```python
from build123d import *

# Parameters (mm, degrees)
SKETCH_1_W      = 68
SKETCH_1_H      = 38
SKETCH_1_R      = 1.5
SKETCH_1_R_2    = 2.5
EXTRUDE_1_DEPTH = 3
SKETCH_2_R      = 4
SKETCH_2_R_2    = 1.5
EXTRUDE_2_DEPTH = 19
FILLET_1_R      = 4


with BuildPart() as part:
    # 草图1 → 凸台-拉伸1 (new body)
    with BuildSketch(Plane(origin=(0, 0, 0), x_dir=(1, 0, 0), z_dir=(0, 1, 0))):
        with Locations((10, -0.865384615)):
            Rectangle(SKETCH_1_W, SKETCH_1_H)
        with Locations(Location((-20, -15.865384615, 0), (0, 0, 270))):
            Circle(SKETCH_1_R, mode=Mode.SUBTRACT)
        with Locations(Location((-20, 14.134615385, 0), (0, 0, 270))):
            Circle(SKETCH_1_R, mode=Mode.SUBTRACT)
        with Locations(Location((40, 14.134615385, 0), (0, 0, 270))):
            Circle(SKETCH_1_R, mode=Mode.SUBTRACT)
        with Locations(Location((40, -15.865384615, 0), (0, 0, 270))):
            Circle(SKETCH_1_R, mode=Mode.SUBTRACT)
        with Locations(Location((-17.5, -0.865384615, 0), (0, 0, 270))):
            Circle(SKETCH_1_R_2, mode=Mode.SUBTRACT)
        with Locations(Location((37.5, -0.865384615, 0), (0, 0, 90))):
            Circle(SKETCH_1_R_2, mode=Mode.SUBTRACT)
        with Locations(Location((25, 14.134615385, 0), (0, 0, 270))):
            Circle(SKETCH_1_R, mode=Mode.SUBTRACT)
    extrude(amount=EXTRUDE_1_DEPTH)

    # 草图2 → 凸台-拉伸2 (add)
    # profile 1 of 4: a face of its own
    with BuildSketch(Plane(origin=(0, 3, 0), x_dir=(1, 0, 0), z_dir=(0, 1, 0))):
        with Locations(Location((-20, -15.865384615, 0), (0, 0, 270))):
            Circle(SKETCH_2_R)
        with Locations(Location((-20, -15.865384615, 0), (0, 0, 270))):
            Circle(SKETCH_2_R_2, mode=Mode.SUBTRACT)
    # profile 2 of 4: a face of its own
    with BuildSketch(Plane(origin=(0, 3, 0), x_dir=(1, 0, 0), z_dir=(0, 1, 0))):
        with Locations(Location((40, -15.865384615, 0), (0, 0, 270))):
            Circle(SKETCH_2_R)
        with Locations(Location((40, -15.865384615, 0), (0, 0, 270))):
            Circle(SKETCH_2_R_2, mode=Mode.SUBTRACT)
    # profile 3 of 4: a face of its own
    with BuildSketch(Plane(origin=(0, 3, 0), x_dir=(1, 0, 0), z_dir=(0, 1, 0))):
        with Locations(Location((-20, 14.134615385, 0), (0, 0, 90))):
            Circle(SKETCH_2_R)
        with Locations(Location((-20, 14.134615385, 0), (0, 0, 270))):
            Circle(SKETCH_2_R_2, mode=Mode.SUBTRACT)
    # profile 4 of 4: a face of its own
    with BuildSketch(Plane(origin=(0, 3, 0), x_dir=(1, 0, 0), z_dir=(0, 1, 0))):
        with Locations(Location((40, 14.134615385, 0), (0, 0, 90))):
            Circle(SKETCH_2_R)
        with Locations(Location((40, 14.134615385, 0), (0, 0, 270))):
            Circle(SKETCH_2_R_2, mode=Mode.SUBTRACT)
    extrude(amount=EXTRUDE_2_DEPTH)

    # 圆角1
    fillet_1_edges = [part.edges().sort_by_distance(p)[0] for p in [
        (44, 1.5, 19.865384615),
        (44, 1.5, -18.134615385),
        (-24, 1.5, -18.134615385),
        (-24, 1.5, 19.865384615),
    ]]
    fillet(fillet_1_edges, radius=FILLET_1_R - 0.0001)  # a hair under: the kernel refuses the full size


solid = part.part
```
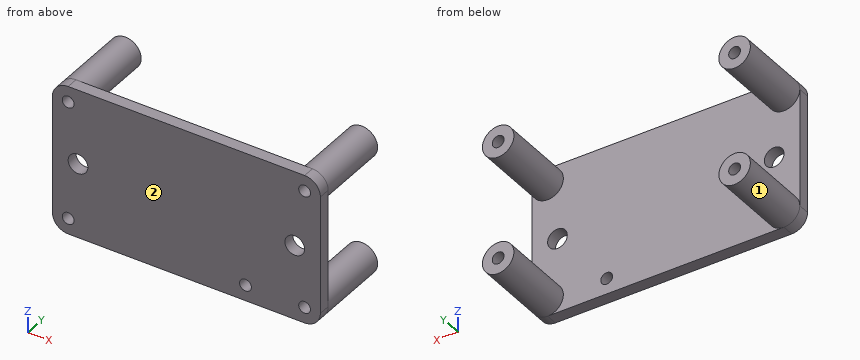
Could you check a few things on this model? Use its own coordinates, in mm. Face numbers are marked on the shaded views. Give positions to 0.01 mm unless a question says otherwise; leave off trailing zeros. Loops run counter-clockwise (first coordinate to the right, second up) from the corner with the lowest first, then second, coordinate; pieces in that order, holes last. Notation, with made-up numbers: (54.25, 84) - (93.25, 84) arc R34 ccw to (93.25, 116) - close; hole circle Ø7 at (84, -20.5). An arc over 180 degrees is marked (long way). Use one line per item in the form item = value.
1. I want a section at D-D (z = 8.5). Please give me the cut outline in (x, y), and give its area (3 significant figures).
Response values:
outline = (-24, 0) - (44, 0) - (44, 3) - (-24, 3) - close
area = 204 mm²
2. I need wall thicknesses on probe 1 along Z at (x, y) = (37.5, 1); probe 2 along Y at (x, z) = (38.5, 11.5); probe 3 along Z at (x, y) = (-18, 6.25). Which ranges of each line are inside material? Lowest first, please.
Response values:
probe_1 = -18.13 to -1.63, 3.37 to 19.87
probe_2 = 0 to 3
probe_3 = -17.6 to -10.67, 12.4 to 19.33
3. I want a section at A-A (y = 15). Please give me the cut outline in (x, z), and give its area (3 significant figures).
Response values:
outline = circle Ø8 at (-20, -14.13); circle Ø8 at (-20, 15.87); circle Ø8 at (40, -14.13); circle Ø8 at (40, 15.87); hole circle Ø3 at (-20, -14.13); hole circle Ø3 at (-20, 15.87); hole circle Ø3 at (40, -14.13); hole circle Ø3 at (40, 15.87)
area = 173 mm²
4. Thinking about a two-plate mould opening in Z: for the marked faces 1 and 2, which applies, released by +Z, released by -Z, zero draft, split by the parting line, or undercut?
Response values:
face_1 = undercut
face_2 = zero draft
5. I'm going to push flat-ended pins straight in: pin 1 Ø2.5 at (x, z) = (40, 15.87) entering from +Y; pin 2 Ø11.5 at (x, z) = (19, 6.5) entering from +Y. Where does each tip first touch, or does it pass through?
Response values:
pin_1 = through
pin_2 = 3
6. I want a section at B-B (x = 25). Please give me the cut outline in (y, z), and give its area (3 significant figures).
Response values:
outline = (0, -18.13) - (3, -18.13) - (3, -15.63) - (0, -15.63) - close; (0, -12.63) - (3, -12.63) - (3, 19.87) - (0, 19.87) - close
area = 105 mm²
7. I want a section at C-C (z = -0.5). Please give me the cut outline in (x, y).
Response values:
outline = (-24, 0) - (-19.59, 0) - (-19.59, 3) - (-24, 3) - close; (-15.41, 0) - (35.41, 0) - (35.41, 3) - (-15.41, 3) - close; (39.59, 0) - (44, 0) - (44, 3) - (39.59, 3) - close
